Verification items for the finished model (mm, model axes). A direction names the side the tool comes from. Coordinates: 2 decimals unless noted, no trailing zeros. Loops run counter-clockwise (first coordinate to the right, second up) from the corner with the lowest first, then second, coordinate; pieces in that order, holes last. Notation, with made-up numbers: M 68.5,9 L 81.5,9 A24 cw 81.5,29 Z; hole C 76.5,48 d7. An arc over 180 degrees is marked long. Write item = value, one per line. Start each with the question number.
```python
from build123d import *

# Parameters (mm, degrees)
IZIM2_R                          = 10.5
Y_KSEKLIK_EKSTR_ZYON1_DEPTH      = 3
Y_KSEKLIK_EKSTR_ZYON3_DEPTH      = 4
Y_KSEKLIK_EKSTR_ZYON3_DEPTH_BACK = 4
Y_KSEKLIK_EKSTR_ZYON6_DEPTH      = 4
Y_KSEKLIK_EKSTR_ZYON6_DEPTH_BACK = 4
IZIM5_W                          = 23.418755165
IZIM5_H                          = 7.378370442
IZIM5_H_2                        = 8.702399003
KES_EKSTR_ZYON1_DEPTH            = 3
IZIM6_W                          = 30
IZIM6_H                          = 8
Y_KSEKLIK_EKSTR_ZYON7_DEPTH      = 17
IZIM7_R                          = 2.5
KES_EKSTR_ZYON2_DEPTH            = 30
IZIM8_R                          = 1.5
KES_EKSTR_ZYON3_DEPTH            = 30
PAH1_SIZE                        = 1.5
PAH2_SIZE                        = 2
IZIM9_R                          = 5.5
KES_EKSTR_ZYON4_DEPTH            = 17


with BuildPart() as part:
    # Çizim2 → Yükseklik-Ekstrüzyon1 (new body)
    with BuildSketch(Plane.XY):
        Circle(IZIM2_R)
    extrude(amount=Y_KSEKLIK_EKSTR_ZYON1_DEPTH)

    # Çizim3 → Yükseklik-Ekstrüzyon3 (add, two sides: drawn at the far end of the back side and taken through both)
    with BuildSketch(Plane(origin=(0, 0, 0), x_dir=(1, 0, 0), z_dir=(0, 1, 0)).offset(-Y_KSEKLIK_EKSTR_ZYON3_DEPTH_BACK)):
        Polygon((-14.349740813, 21.832604096), (0, 4.731248928), (14.349740813, 21.832604096), (3.3694522, 37.514081392), (3.3694522, 44.514081392), (20.58445702, 19.928506573), (3.862454505, 0), (-3.862454505, 0), (-20.58445702, 19.928506573), (-3.3694522, 44.514081392), (-3.3694522, 37.514081392), align=None)
    extrude(amount=Y_KSEKLIK_EKSTR_ZYON3_DEPTH + Y_KSEKLIK_EKSTR_ZYON3_DEPTH_BACK)

    # Çizim4 → Yükseklik-Ekstrüzyon6 (add, two sides: drawn at the far end of the back side and taken through both)
    with BuildSketch(Plane(origin=(0, 0, 0), x_dir=(0, 0, -1), z_dir=(1, 0, 0)).offset(-Y_KSEKLIK_EKSTR_ZYON6_DEPTH_BACK)):
        Polygon((44.514081392, 6.527514275), (37.514081392, 6.527514275), (19.878054627, 16.709679075), (4.731248928, 4), (4.731248928, -4), (19.878054627, -16.709679075), (37.514081392, -6.527514275), (44.514081392, -6.527514275), (19.928506573, -20.722002515), (0, -4), (0, 4), (19.928506573, 20.722002515), align=None)
    extrude(amount=Y_KSEKLIK_EKSTR_ZYON6_DEPTH + Y_KSEKLIK_EKSTR_ZYON6_DEPTH_BACK)

    # Çizim5 → Kes-Ekstrüzyon1 (cut)
    with BuildSketch(Plane.XY.offset(3)):
        with Locations((0.537886602, 7.689185221)):
            Rectangle(IZIM5_W, IZIM5_H)
        with Locations((0.537886602, -8.351199502)):
            Rectangle(IZIM5_W, IZIM5_H_2)
    extrude(amount=-KES_EKSTR_ZYON1_DEPTH, mode=Mode.SUBTRACT)

    # Çizim6 → Yükseklik-Ekstrüzyon7 (add)
    with BuildSketch(Plane.XY.offset(3)):
        Rectangle(IZIM6_W, IZIM6_H)
    extrude(amount=Y_KSEKLIK_EKSTR_ZYON7_DEPTH)

    # Çizim7 → Kes-Ekstrüzyon2 (cut)
    with BuildSketch(Plane(origin=(15, 0, 0), x_dir=(0, 0, -1), z_dir=(1, 0, 0))):
        with Locations(Location((-15, 0, 0), (0, 0, 90))):
            Circle(IZIM7_R)
    extrude(amount=-KES_EKSTR_ZYON2_DEPTH, mode=Mode.SUBTRACT)

    # Çizim8 → Kes-Ekstrüzyon3 (cut)
    with BuildSketch(Plane.ZY.offset(15)):
        with Locations(Location((7, 0, 0), (0, 0, 270))):
            Circle(IZIM8_R)
    extrude(amount=-KES_EKSTR_ZYON3_DEPTH, mode=Mode.SUBTRACT)

    # Pah1
    pah1_edges = [part.edges().sort_by_distance(p)[0] for p in [
        (15, -4, 11.5),
        (15, 4, 11.5),
        (-15, -4, 11.5),
        (-15, 4, 11.5),
    ]]
    chamfer(pah1_edges, length=PAH1_SIZE - 0.0001)  # a hair under: the kernel refuses the full size

    # Pah2
    pah2_edges = [part.edges().sort_by_distance(p)[0] for p in [
        (15, 0, 3),
        (-15, 0, 3),
    ]]
    chamfer(pah2_edges, length=PAH2_SIZE)

    # Çizim9 → Kes-Ekstrüzyon4 (cut)
    with BuildSketch(Plane(origin=(0, 4, 0), x_dir=(1, 0, 0), z_dir=(0, 1, 0))):
        with Locations(Location((0, -10, 0), (0, 0, 270))):
            Circle(IZIM9_R)
    extrude(amount=-KES_EKSTR_ZYON4_DEPTH, mode=Mode.SUBTRACT)


solid = part.part
```
Q1. Sectioned sample at B-B on x = -1.5. Record the cut outline in (y, z), plus the area to 3 significant figures.
Q2. Sectioned sample at D-D on z = -26.5. Record the cut outline in (x, y), plus the area to 3 significant figures.
Q3. Set-up check for faces 1 (the face through (10.5, -0.1, 1.5)), 2 (the face through (-0.056, 10.444, -12.411)), 3 (the face through (-3.369, 0, -41)), 4 (the face through (0, -6.528, -41)): record each of +Z, -Z, +X, -X, +Y, -Y from which the full face is reachable in a straight line by a thin tool's end or side.
Q4. Sectioned sample at A-A on z = 10. Record the cut outline in (x, y).
Q5. Gauge pin test, flat ends, axial feed: pin 1 (3 mm diameter, centred on x = -4.5, z = -32.5, fed in from +Y); pin 2 (5 mm diameter, centred on y = 0, z = 7, fed in from +X); pin 3 (16 mm diameter, centred on x = 0, z = 6.5, fed in from -Y). Record the tip position at first contact, or that the pin passes through.
Q6. Mould release check, pull along Z, two halves, no side actions. Record for faces 5 (the face through (11.86, -0.06, -32.39)), 6 (the face through (0, 0, 20)), 7 (the face through (7.07, -0.06, -13.16)), 8 (the face through (-14, 0, 4)): +Z half, -Z half, draft (parallel to the pull), parting line (faces both ways), or undercut.
Q7. Sectioned sample at C-C on y = -9. Record the cut outline in (x, z), plus the area to 4 significant figures.
Q8. Scan lines: L1, parallel to X at y = -1.5, z = 10; L2, parallel to Z at x = -5.75, y = 0; L3, parallel to Z at x = -6, y = 0. Record each from-to range of solid material in increasing order. Write a range as [from, to].
Solutions:
q1.outline = M -20.72,-19.93 L -6.53,-44.51 L -6.53,-37.51 L -16.71,-19.88 L -4,-4.73 L -4,-6.52 L 4,-6.52 L 4,-4.73 L 16.71,-19.88 L 6.53,-37.51 L 6.53,-44.51 L 20.72,-19.93 L 4,0 L 4,4.71 L -4,4.71 L -4,0 Z; M -4,15.29 L -2.48,15.29 A2.5 cw 2.48,15.29 L 4,15.29 L 4,20 L -4,20 Z
q1.area = 429 mm²
q2.outline = M -15.98,-4 L -11.08,-4 L -11.08,4 L -15.98,4 Z; M -4,-16.93 L 4,-16.93 L 4,-12.89 L -4,-12.89 Z; M -4,12.89 L 4,12.89 L 4,16.93 L -4,16.93 Z; M 11.08,-4 L 15.98,-4 L 15.98,4 L 11.08,4 Z
q2.area = 143 mm²
q3.face_1 = +X
q3.face_2 = +X, -X
q3.face_3 = -Z
q3.face_4 = -Z, +X, -X
q4.outline = M -15,-2.5 L -13.5,-4 L -5.5,-4 L -5.5,4 L -13.5,4 L -15,2.5 Z; M 5.5,-4 L 13.5,-4 L 15,-2.5 L 15,2.5 L 13.5,4 L 5.5,4 Z
q5.pin_1 = 14.28
q5.pin_2 = 15
q5.pin_3 = -5.26
q6.face_5 = -Z half
q6.face_6 = +Z half
q6.face_7 = undercut
q6.face_8 = undercut
q7.outline = M -4,-40.23 L 4,-40.23 L 4,-33.23 L -4,-33.23 Z; M -4,-10.69 L 4,-10.69 L 4,-5.96 L -4,-5.96 Z
q7.area = 93.85 mm²
q8.L1 = [-15, -5.5], [5.5, 15]
q8.L2 = [-41.11, -34.11], [-11.58, -2.25], [0, 5.5], [8.5, 12.5], [17.5, 20]
q8.L3 = [-40.76, -33.76], [-11.88, -2.55], [0, 5.5], [8.5, 12.5], [17.5, 20]
